Verification items for the finished model (mm, model axes). Face numbers are marked on the shaded views. Coordinates: 2 decimals unless noted, no trailing zeros. Loops run counter-clockwise (first coordinate to the right, second up) from the corner with the lowest first, then second, coordinate; pieces in that order, holes last. Notation, with made-up numbers: (-18, 52.5) -> (-9, 52.5) arc R17 ccw to (-9, 76.5) -> close; hole circle Ø6 at (65.25, 65). An arc over 180 degrees is marked (long way). Answer as a JSON object with one key per item and string values. Group by question number.
Q1. Release check for a two-part mould opening along X. For the marked faces 1, 2 and 3 record: released by +X, released by -X, zero draft, split by the parting line, or undercut.
Q2. Cross-section at C-C on z = 18.5. Record the boundary of the cut face in (x, y).
Q3. Cross-section at A-A on y = 0. Record the boundary of the cut face in (x, z), and give its area (3 significant figures).
Q4. Scan lines: L1, parallel to Y at x = 0, z = 6; L2, parallel to Y at x = -1.5, z = 7.5; L3, parallel to X at y = -14, z = 27.25. Record each from-to range of solid material in increasing order.
Q5. Cross-section at B-B on x = 0. Record the boundary of the cut face in (y, z).
Q6. Cross-section at D-D on y = 7. Record the boundary of the cut face in (x, z).
Q7. Gauge pin test, flat ends, axial feed: pin 1 Ø3 at (y, z) = (-19, 10) entering from +X; pin 2 Ø3 at (x, z) = (-17.5, 25.5) entering from +Y; pin 3 Ø1 at (x, z) = (0, 6) entering from -Y. Record the tip position at first contact, or that the pin passes through.
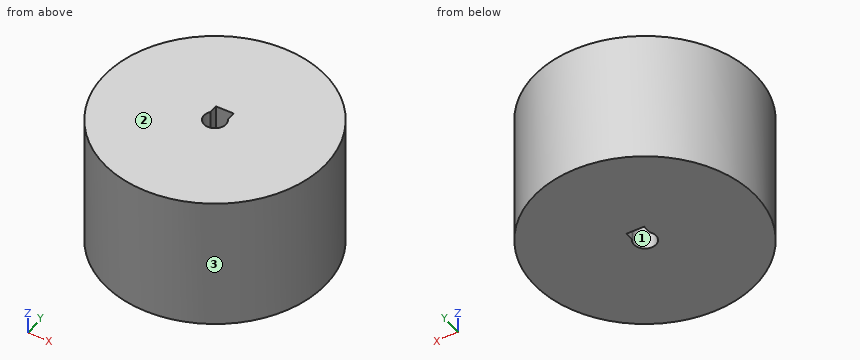
```python
from build123d import *

# Parameters (mm, degrees)
ESQUISSE1_R             = 25
BOSS_EXTRU_1_DEPTH      = 30
ESQUISSE14_R            = 2.5
ENL_V_MAT_EXTRU_1_DEPTH = 47.368092477
ESQUISSE15_W            = 4
ESQUISSE15_H            = 2
ENL_V_MAT_EXTRU_2_DEPTH = 47.368092477


with BuildPart() as part:
    # Esquisse1 → Boss.-Extru.1 (new body)
    with BuildSketch(Plane.XY):
        Circle(ESQUISSE1_R)
    extrude(amount=BOSS_EXTRU_1_DEPTH)

    # Esquisse14 → Enlèv. mat.-Extru.1 (cut, through all)
    with BuildSketch(Plane(origin=(0, 0, 0), x_dir=(-1, 0, 0), z_dir=(0, 0, -1))):
        Circle(ESQUISSE14_R)
    extrude(amount=-ENL_V_MAT_EXTRU_1_DEPTH, mode=Mode.SUBTRACT)

    # Esquisse15 → Enlèv. mat.-Extru.2 (cut, through all)
    with BuildSketch(Plane(origin=(0, 0, 0), x_dir=(-1, 0, 0), z_dir=(0, 0, -1))):
        with Locations((0, 2.5)):
            Rectangle(ESQUISSE15_W, ESQUISSE15_H)
    extrude(amount=-ENL_V_MAT_EXTRU_2_DEPTH, mode=Mode.SUBTRACT)


solid = part.part
```
Computed values:
{
 "1": {"face 1": "undercut", "face 2": "zero draft", "face 3": "split by the parting line"},
 "2": {"outline": "circle Ø50 at (0, 0); hole (-2, 1.5) arc R2.5 ccw (long way) to (2, 1.5) -> (2, 3.5) -> (-2, 3.5) -> close"},
 "3": {"outline": "(-25, 0) -> (-2.5, 0) -> (-2.5, 30) -> (-25, 30) -> close; (2.5, 0) -> (25, 0) -> (25, 30) -> (2.5, 30) -> close", "area": "1,350 mm²"},
 "4": {"L1": "y = -25 to -2.5, 3.5 to 25", "L2": "y = -24.95 to -2, 3.5 to 24.95", "L3": "x = -20.71 to 20.71"},
 "5": {"outline": "(-25, 0) -> (-2.5, 0) -> (-2.5, 30) -> (-25, 30) -> close; (3.5, 0) -> (25, 0) -> (25, 30) -> (3.5, 30) -> close"},
 "6": {"outline": "(-24, 0) -> (24, 0) -> (24, 30) -> (-24, 30) -> close"},
 "7": {"pin 1": "stops at x = 17.85", "pin 2": "stops at y = 19.21", "pin 3": "stops at y = -25"}
}
